Autodesk Inventor part; units mm, degrees
ref_plane "YZ Plane" through (0, 0, 0) normal (1, 0, 0) x (0, 1, 0)
ref_plane "XZ Plane" through (0, 0, 0) normal (0, 1, 0) x (-1, 0, 0)
ref_plane "XY Plane" through (0, 0, 0) normal (0, 0, 1) x (1, 0, 0)
sketch "スケッチ1" plane through (0, 0, 0) normal (0, 0, 1) x (1, 0, 0)
  line L0 (0, 0) -> (9, 0)
  line L1 (9, 0) -> (9, -9)
  line L2 (9, -9) -> (0, -9)
  line L3 (0, -9) -> (0, 0)
  line L4 (1.2, -1.2) -> (7.8, -1.2)
  line L5 (7.8, -1.2) -> (7.8, -7.8)
  line L6 (7.8, -7.8) -> (1.2, -7.8)
  line L7 (1.2, -7.8) -> (1.2, -1.2)
  dimension "d0" = 9
  dimension "d1" = 9
  dimension "d2" = 6.6
  dimension "d3" = 6.6
  dimension "d4" = 1.2
  dimension "d5" = 1.2
extrude "押し出し1" add sketch "スケッチ1" along normal blind 80
sketch "スケッチ2" plane through (9, -9, 0) normal (1, 0, 0) x (0, 0, -1)
  line L0 (0, 9) -> (-80, 9)
  line L1 (-80, 0) -> (-80, 9)
  line L2 (0, 0) -> (0, 9)
  point P0 (-41, 4.5)
  point P1 (-25, 4.5)
  dimension "d8" = 16
  dimension "d9" = 4.5
  dimension "d10" = 4.5
  dimension "d11" = 80
  dimension "d42" = 25
hole "穴1" at (9, -4.5, 41) at (9, -4.5, 25) direction (-1, 0, 0) diameter 3 end through all
sketch "スケッチ3" plane through (0, -9, 0) normal (0, -1, 0) x (1, 0, 0)
  line L0 (0, 80) -> (9, 80)
  line L1 (0, 0) -> (9, 0)
  line L2 (9, 0) -> (9, 80)
  point P0 (4.5, 4.5)
  point P1 (4.5, 75.5)
  dimension "d20" = 4.5
  dimension "d21" = 4.5
  dimension "d22" = 4.5
  dimension "d23" = 4.5
hole "穴2" at (4.5, -9, 4.5) at (4.5, -9, 75.5) direction (0, 1, 0) diameter 3 end through all
sketch "スケッチ4" plane through (9, -9, 0) normal (1, 0, 0) x (0, 0, -1)
  line L0 (0, 0) -> (0, 9)
  line L1 (-80, 0) -> (-80, 9)
  line L2 (0, 0) -> (-80, 0)
  point P0 (-13.5, 4.5)
  point P1 (-66.5, 4.5)
  dimension "d31" = 13.5
  dimension "d32" = 13.5
  dimension "d33" = 4.5
  dimension "d34" = 4.5
hole "穴3" at (9, -4.5, 13.5) at (9, -4.5, 66.5) direction (-1, 0, 0) diameter 3 end through all
sketch "スケッチ5" plane through (0, -9, 0) normal (0, -1, 0) x (1, 0, 0)
  line L0 (0, 0) -> (0, 80)
  circle A0 centre (4.5, 4.5) radius 1.5
  point P0 (4.5, 11.5)
  point P1 (4.5, 18.5)
  point P2 (4.5, 25.5)
  point P3 (4.5, 32.5)
  point P4 (4.5, 39.5)
  point P5 (4.5, 46.5)
  point P6 (4.5, 53.5)
  point P7 (4.5, 60.5)
  point P8 (4.5, 67.5)
  dimension "d43" = 4.5
  dimension "d44" = 7
  dimension "d47" = 7
hole "穴4" at (4.5, -9, 11.5) at (4.5, -9, 18.5) at (4.5, -9, 25.5) at (4.5, -9, 32.5) at (4.5, -9, 39.5) at (4.5, -9, 46.5) at (4.5, -9, 53.5) at (4.5, -9, 60.5) at (4.5, -9, 67.5) direction (0, 1, 0) diameter 6 end through all
properties part number "上下直動9x9_1" material "アルミニウム 6061"
Read the model definition and answer for the solid it produces. Units are mm, in the model's axes. A direction names the side the tool comes from. Give positions to 0.01 mm unless a question says otherwise; leave off trailing zeros. Loops run counter-clockwise (first coordinate to the right, second up) from the corner with the lowest first, then second, coordinate; pieces in that order, holes last. Notation, with made-up numbers: (67, 63.5) -> (78, 63.5) arc R22 cw to (78, 86.5) -> close; hole circle Ø10 at (84.5, 32.25). An arc over 180 degrees is marked (long way). Answer as CSV lines item,"result".
Item 1: Find section D-D on x = 6.75. State how many separate pieces and enclosed holes the cut face has, plus the area to 3 significant figures.
Returned:
separate pieces,"20"
enclosed holes,"0"
area,"106 mm²"
Item 2: Consider line 1 (X direction, y = -6, z = 40); line 2 (X direction, y = -8.65, z = 60.5); line 3 (Y direction, x = 6.5, z = 50). Determine where each line is inside the solid, lowest interval first. Write a range as [from, to].
Returned:
line 1,"x = [0, 1.2], [7.8, 9]"
line 2,"x = [0, 1.5], [7.5, 9]"
line 3,"y = [-9, -7.8], [-1.2, 0]"
Item 3: Determine the mould class of faces 3 (the face through (8, -9, 39)), 4 (the face through (4.4, -0.6, 42.5)) for opening direction Z: +Z half, -Z half, draft (parallel to the pull), parting line (faces both ways), or undercut.
Returned:
face 3,"draft"
face 4,"undercut"
Item 4: Find section B-B on y = -7. Give the vertices of the cut face in (x, z).
Returned:
outline,"(0, 0) -> (1.2, 0) -> (1.2, 80) -> (0, 80) -> close; (7.8, 0) -> (9, 0) -> (9, 80) -> (7.8, 80) -> close"
Item 5: For faces 1 (the face through (2.47, -0.59, 27.71)), 2 (the face through (1.5, -1.2, 30.6)), determine the directions among +Z, -Z, +X, -X, +Y, -Y from which every point of the face is accessible in a straight line to the end or side of a thin tool.
Returned:
face 1,"+Y, -Y"
face 2,"+Z, -Z"
Item 6: Find section A-A on z = 53.5. Give the vertices of the cut face in (x, y).
Returned:
outline,"(0, -9) -> (1.5, -9) -> (1.5, -7.8) -> (1.2, -7.8) -> (1.2, -1.2) -> (1.5, -1.2) -> (1.5, 0) -> (0, 0) -> close; (7.5, -9) -> (9, -9) -> (9, 0) -> (7.5, 0) -> (7.5, -1.2) -> (7.8, -1.2) -> (7.8, -7.8) -> (7.5, -7.8) -> close"
Item 7: Find section C-C on z = 7. Give the vertices of the cut face in (x, y).
Returned:
outline,"(0, -9) -> (9, -9) -> (9, 0) -> (0, 0) -> close; hole (1.2, -7.8) -> (7.8, -7.8) -> (7.8, -1.2) -> (1.2, -1.2) -> close"
Item 8: This flat-tipped pin is pushed along its axis until it touches: pin 1 (5 mm diameter, centred on y = -4.5, z = 25, fed in from -X). Where does it stop, or does it pass through?
Returned:
pin 1,"stops at x = 0"
